Here's how the part is built. I have some questions about the finished solid (model axes, mm). A direction names the side the tool comes from. Give positions to 0.01 mm unless a question says otherwise; leave off trailing zeros. Loops run counter-clockwise (first coordinate to the right, second up) from the corner with the lowest first, then second, coordinate; pieces in that order, holes last.
Q1. Thinking about a two-plate mould opening in Y: for faces 1 (the face through (-6, 4.05, 2)), 2 (the face through (-5.48, 3.9, -7.14)), 3 (the face through (-2.681, 0.043, 6.466)), which applies, pulls with the +Y half, pulls with the -Y half, needs draft (parallel to the pull), parting line crosses it, or undercut?
Q2. Suppose I cut it at B-B (x = 0). List the corners of the cut face in (y, z) for me (3 decimals).
Q3. I'm going to push flat-ended pins straight in: P1, Ø1, axis at x = -6.5, y = 0, coming from the +Z side; P2, Ø3, axis at y = 3, z = 1.5, coming from the +X side. Where does each tip first touch, or does it pass through?
Q4. Suppose I cut it at C-C (y = 2.75). List the corners of the cut face in (x, z) for me (3 decimals), and give its area (3 significant figures).
Q5. I need wall thicknesses on probe 1 along Y at (x, z) = (7, -3); probe 2 along X at (y, z) = (1, 0) (3 decimals); probe 3 along X at (y, z) = (-1, 3.25). Which ranges of each line are inside material? Lowest first, please.
Q6. Suppose I cut it at A-A (z = 0). List the corners of the cut face in (x, y) for me (3 decimals), and give its area (3 significant figures).
Q7. For faces 4 (the face through (-6, -4.05, 2)), 5 (the face through (3.8, 3.25, -6.3)), which set-ups out of +Z, -Z, +X, -X, +Y, -Y let a thin tool reach every point of the face, with its end or its side?
Autodesk Inventor part; units mm, degrees
ref_plane "YZ Plane" through (0, 0, 0) normal (1, 0, 0) x (0, 1, 0)
ref_plane "XZ Plane" through (0, 0, 0) normal (0, 1, 0) x (-1, 0, 0)
ref_plane "XY Plane" through (0, 0, 0) normal (0, 0, 1) x (1, 0, 0)
sketch "Esboço1" plane through (0, 0, 0) normal (1, 0, 0) x (0, 1, 0)
  line L0 (-4.05, 9) -> (-3.25, 9)
  line L1 (-3.25, 9) -> (-3.25, 7)
  line L2 (-3.25, 7) -> (3.25, 7)
  line L3 (3.25, 7) -> (3.25, 9)
  line L4 (3.25, 9) -> (4.05, 9)
  line L5 (4.05, 9) -> (4.05, 5.475)
  line L6 (-2.5, 5.475) -> (-4.05, 5.475)
  line L7 (-4.05, 5.475) -> (-4.05, 9)
  line L8 (-21.75, 0) -> (21.75, 0)
  line L9 (-2.5, 5.475) -> (-2.5, 5.475)
  line L10 (2.5, 5.475) -> (2.5, 5.475)
  line L11 (2.5, 5.475) -> (3.5, 5.475)
  line L12 (3.5, 5.475) -> (3.5, 5.475)
  line L13 (4.05, 5.475) -> (3.5, 5.475)
  line L14 (2.5, 5.475) -> (-2.5, 5.475)
  point P0 (0, 0)
  point P1 (0, 0)
  point P2 (0, 5.475)
  point P3 (0, 7)
  dimension "d3" = 0.8
  dimension "d4" = 14
  dimension "d5" = 18
  dimension "d11" = 2.5
  dimension "d14" = 10.95
  dimension "d16" = 6.5
  dimension "d17" = 2.5
  dimension "d19" = 10.95
  dimension "d20" = 125
  dimension "d21" = 0
  dimension "d22" = 1
revolve "Revolução1" add sketch "Esboço1" angle 360 about axis through (0, -21.75, 0) along (0, 1, 0)
fillet "Arredondamento1" radius 0.2 2 edges at (0, 3.25, -7) (0, -3.25, -7)
chamfer "Chamfer2" distance 0.5 angle 45 2 edges at (0, -3.25, -9) (0, 3.25, -9)
chamfer "Chamfer3" distance 0.5 angle 45 2 edges at (0, -4.05, -5.475) (0, 4.05, -5.475)
properties part number "PoliaLisaGT2" material "Aluminum 6061"
Solutions:
1. face 1: pulls with the +Y half
1. face 2: needs draft
1. face 3: undercut
2. outline: (-4.05, -9) - (-3.75, -9) - (-3.25, -8.5) - (-3.25, -7.2) arc R0.2 cw to (-3.05, -7) - (3.05, -7) arc R0.2 cw to (3.25, -7.2) - (3.25, -8.5) - (3.75, -9) - (4.05, -9) - (4.05, -5.975) - (3.55, -5.475) - (-3.55, -5.475) - (-4.05, -5.975) - close; (-4.05, 5.975) - (-3.55, 5.475) - (3.55, 5.475) - (4.05, 5.975) - (4.05, 9) - (3.75, 9) - (3.25, 8.5) - (3.25, 7.2) arc R0.2 cw to (3.05, 7) - (-3.05, 7) arc R0.2 cw to (-3.25, 7.2) - (-3.25, 8.5) - (-3.75, 9) - (-4.05, 9) - close
3. P1: stops at z = 3.61
3. P2: stops at x = 9
4. outline: circle Ø14 at (0, 0); hole circle Ø10.95 at (0, 0)
4. area: 59.8 mm2
5. probe 1: y = -4.05 to -3.25, 3.25 to 4.05
5. probe 2: x = -7 to -5.475, 5.475 to 7
5. probe 3: x = -6.2 to -4.41, 4.41 to 6.2
6. outline: (-9, -4.05) - (-5.975, -4.05) - (-5.475, -3.55) - (-5.475, 3.55) - (-5.975, 4.05) - (-9, 4.05) - (-9, 3.75) - (-8.5, 3.25) - (-7.2, 3.25) arc R0.2 cw to (-7, 3.05) - (-7, -3.05) arc R0.2 cw to (-7.2, -3.25) - (-8.5, -3.25) - (-9, -3.75) - close; (5.475, -3.55) - (5.975, -4.05) - (9, -4.05) - (9, -3.75) - (8.5, -3.25) - (7.2, -3.25) arc R0.2 cw to (7, -3.05) - (7, 3.05) arc R0.2 cw to (7.2, 3.25) - (8.5, 3.25) - (9, 3.75) - (9, 4.05) - (5.975, 4.05) - (5.475, 3.55) - close
6. area: 30.1 mm2
7. face 4: +Z, -Z, +X, -X, -Y
7. face 5: none
